from build123d import *

# Parameters (mm, degrees)
F0_W     = 177
F0_H     = 85
F1_DEPTH = 17.4
F2_W     = 172
F2_H     = 2.7
F3_DEPTH = 9.7


with BuildPart() as f1:
    # F0 (on Top) → F1 (new body)
    with BuildSketch(Plane.XY):
        Rectangle(F0_W, F0_H)
    extrude(amount=F1_DEPTH)

    # F2 (on face) → F3 (cut)
    with BuildSketch(Plane.XY.offset(17.4)):
        Rectangle(F2_W, F2_H)
    extrude(amount=-F3_DEPTH, mode=Mode.SUBTRACT)


solid = f1.part
The listing builds one solid part. Answer for the finished solid, in the listing's coordinates (mm). A direction names the side the tool comes from. Round coordinates to 2 decimals unless told otherwise and drop trailing zeros. Loops run counter-clockwise (first coordinate to the right, second up) from the corner with the lowest first, then second, coordinate; pieces in that order, holes last. Notation, with made-up numbers: M 16,38.5 L 46,38.5 A19 ccw 46,42.5 Z; hole C -1,85 d7. An arc over 180 degrees is marked long. Write each question's results on one line, items separated by ' | '. Start each with the question number.
1) Find section B-B on x = 30.5. Write down the section's boundary in (y, z).
2) Which of the six approach directions +Z, -Z, +X, -X, +Y, -Y give full straight-line access (tool end or side, diameter ignored) to faces 1 (the flat face through (-1, -1.35, 13)), 2 (the flat face through (-1, 1, 0))?
3) This flat-tipped pin is pushed along its axis until it touches: pin 1 (3 mm diameter, centred on x = -9, y = 0, fed in from +Z). Where does it stop, or does it pass through?
4) Find section A-A on z = 15.5. Write down the section's boundary in (x, y), plus the area to 3 significant figures.
5) Determine the mould class of faces 3 (the flat face through (-88.5, -1, 9)), 4 (the flat face through (88.5, -1, 9)), 5 (the flat face through (-1, 1.35, 13)) for opening direction X: pulls with the +X half, pulls with the -X half, needs draft (parallel to the pull), parting line crosses it, or undercut.
6) Straight lines are drawn through the part: probe 1 along Y at (x, z) = (30.5, 16); probe 2 along X at (y, z) = (0.5, 15.5); probe 3 along Z at (x, y) = (-69, 1). For each, find the intervals that lie inside material, in ascending order.
Final values:
1) outline: M -42.5,0 L 42.5,0 L 42.5,17.4 L 1.35,17.4 L 1.35,7.7 L -1.35,7.7 L -1.35,17.4 L -42.5,17.4 Z
2) face 1: +Z | face 2: -Z, +X, -X, +Y, -Y
3) pin 1: z = 17.4
4) outline: M -88.5,-42.5 L 88.5,-42.5 L 88.5,42.5 L -88.5,42.5 Z; hole M -86,-1.35 L 86,-1.35 L 86,1.35 L -86,1.35 Z | area: 14,600 mm²
5) face 3: pulls with the -X half | face 4: pulls with the +X half | face 5: undercut
6) probe 1: -42.5 to -1.35, 1.35 to 42.5 | probe 2: -88.5 to -86, 86 to 88.5 | probe 3: 0 to 7.7
